Model file for the job. Use its own axes, mm. Face numbers are marked on the shaded views. A direction names the side the tool comes from. Round coordinates to 2 decimals unless told otherwise and drop trailing zeros. Order: outer loops, then holes, each group sorted by start corner. A loop starts at its lowest first (then second) coordinate and runs counter-clockwise, first axis right, second up. Notation, with made-up numbers: (6, 70.5) - (36, 70.5) arc R8 cw to (36, 78.5) - close; hole circle Ø9 at (8.5, 76.25). An arc over 180 degrees is marked (long way). Put each result on its own line as item: value. Start each with the question number.
Item 1: Saw through at A-A on z = -3.5. List the corners of the cut face in (x, y), plus the area to 3 significant figures.
Item 2: Pin check, flat tips, straight feed: pin 1 Ø3 at (x, y) = (17.51, 2.54) entering from -Z; pin 2 Ø1.5 at (x, y) = (-4.5, 4) entering from +Z; pin 3 Ø3.5 at (x, y) = (16, 3) entering from -Z; pin 4 Ø0.7 at (y, z) = (9.5, -3) entering from +X. Stop position of each tip, or through.
Item 3: Probe probe 1 along X at (y, z) = (9.5, -6.25); probe 2 along X at (y, z) = (9, -3.25); probe 3 along Y at (x, z) = (9, 1). List the from-to ranges inside material, lowest first.
Item 4: Mould opens along Y. For the marked faces 6, 7 and 8 say: pulls with the +Y half, pulls with the -Y half, needs draft (parallel to the pull), parting line crosses it, or undercut.
Item 5: Saw through at C-C on z = 4. List the corners of the cut face in (x, y), plus the area to 3 significant figures.
Item 6: Which spindle directions (+Z, -Z, +X, -X, +Y, -Y) get a long thin tool onto all of the face, cutting with end or side? Do the marked faces 1, 2, 3, 4 and 5. Say none if no direction does.
Item 7: Saw through at B-B on x = 6.5. List the corners of the cut face in (y, z).
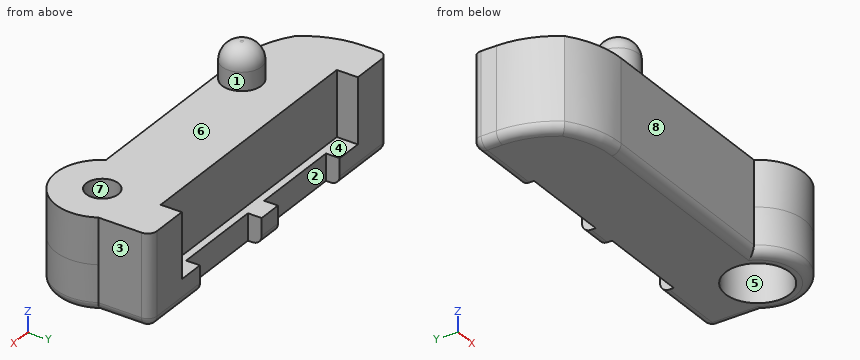
```python
from build123d import *

# Parameters (mm, degrees)
CROQUIS1_W              = 33
CROQUIS1_H              = 5
SALIENTE_EXTRUIR1_DEPTH = 8.5
CROQUIS2_W              = 5
CROQUIS2_H              = 8.5
SALIENTE_EXTRUIR2_DEPTH = 14
CORTAR_EXTRUIR1_REACH   = 34.055
CROQUIS5_R              = 5.070689822
SALIENTE_EXTRUIR3_DEPTH = 5
CROQUIS6_R              = 1.75
CORTAR_EXTRUIR2_DEPTH   = 5
SALIENTE_EXTRUIR4_START = 5
CROQUIS7_R              = 3.5
SALIENTE_EXTRUIR4_DEPTH = 5
SALIENTE_EXTRUIR5_DEPTH = 2.3
CROQUIS9_W              = 10
CROQUIS9_H              = 2.9
CORTAR_EXTRUIR3_DEPTH   = 1.5
CHAFL_N1_SIZE           = 4
REDONDEO1_R             = 10
REDONDEO3_R             = 1
REDONDEO4_R             = 1
REDONDEO5_R             = 1
REDONDEO6_R             = 1
REDONDEO7_R             = 1
CROQUIS10_R             = 2.15
SALIENTE_EXTRUIR6_DEPTH = 4
REDONDEO8_R             = 2


with BuildPart() as part:
    # Croquis1 → Saliente-Extruir1 (new body)
    with BuildSketch(Plane(origin=(0, 0, 0), x_dir=(1, 0, 0), z_dir=(0, 1, 0))):
        Rectangle(CROQUIS1_W, CROQUIS1_H)
    extrude(amount=SALIENTE_EXTRUIR1_DEPTH)

    # Croquis2 → Saliente-Extruir2 (add)
    with BuildSketch(Plane(origin=(16.5, 0, 0), x_dir=(0, 0, -1), z_dir=(1, 0, 0))):
        with Locations((0, 4.25)):
            Rectangle(CROQUIS2_W, CROQUIS2_H)
    extrude(amount=SALIENTE_EXTRUIR2_DEPTH)

    # Croquis4 → Cortar-Extruir1 (cut, up to next)
    with BuildSketch(Plane(origin=(0, 0, -2.5), x_dir=(-1, 0, 0), z_dir=(0, 0, -1)), mode=Mode.PRIVATE) as cortar_extruir1_sk1:
        Polygon((-21.898835729, 8.5), (-21.898835729, 2.753380039), (-21.898835729, 0), (-30.5, 0), (-30.5, 8.5), align=None)
    cortar_extruir1_tool1 = extrude(cortar_extruir1_sk1.sketch, amount=-CORTAR_EXTRUIR1_REACH, mode=Mode.PRIVATE) & part.part
    add(cortar_extruir1_tool1.solids().sort_by_distance((26.199418, 4.25, -2.5))[0], mode=Mode.SUBTRACT)

    # Croquis5 → Saliente-Extruir3 (add)
    with BuildSketch(Plane(origin=(0, 0, -2.5), x_dir=(-1, 0, 0), z_dir=(0, 0, -1))):
        with Locations((-17.511321809, 2.541971061)):
            Circle(CROQUIS5_R)
    extrude(amount=-SALIENTE_EXTRUIR3_DEPTH)

    # Croquis6 → Cortar-Extruir2 (cut)
    with BuildSketch(Plane(origin=(0, 0, -2.5), x_dir=(-1, 0, 0), z_dir=(0, 0, -1))):
        with Locations((-17.511321809, 2.541971061)):
            Circle(CROQUIS6_R)
    extrude(amount=-CORTAR_EXTRUIR2_DEPTH, mode=Mode.SUBTRACT)

    # Croquis7 → Saliente-Extruir4 (add)
    with BuildSketch(Plane(origin=(0, 0, -2.5), x_dir=(-1, 0, 0), z_dir=(0, 0, -1)).offset(SALIENTE_EXTRUIR4_START)):
        with BuildLine():
            Line((-21.898835729, 8.5), (-21.898835729, 5.083942123))
            ThreePointArc((-21.898835729, 5.083942123), (-20.05329287, -1.845542858), (-13.123807889, 0))
            Line((-13.123807889, 0), (16.5, 0))
            Line((16.5, 0), (16.5, 8.5))
            Line((16.5, 8.5), (-21.898835729, 8.5))
        make_face()
        with Locations((-17.511321809, 2.541971061)):
            Circle(CROQUIS7_R, mode=Mode.SUBTRACT)
    extrude(amount=-SALIENTE_EXTRUIR4_DEPTH)

    # Croquis8 → Saliente-Extruir5 (add)
    with BuildSketch(Plane(origin=(0, 8.5, 0), x_dir=(1, 0, 0), z_dir=(0, 1, 0))):
        Polygon((-16.5, -2.5), (-11.620504371, -2.5), (-11.620504371, -2.1), (-11.620504371, 4.6), (16.879495629, 4.6), (16.879495629, -2.1), (16.879495629, -2.5), (21.898835729, -2.5), (21.898835729, 7.5), (-16.5, 7.5), align=None)
    extrude(amount=SALIENTE_EXTRUIR5_DEPTH)

    # Croquis9 → Cortar-Extruir3 (cut)
    with BuildSketch(Plane(origin=(0, 10.8, 0), x_dir=(1, 0, 0), z_dir=(0, 1, 0))):
        with Locations((8.949495629, 6.05)):
            Rectangle(CROQUIS9_W, CROQUIS9_H)
        with Locations((-3.690504371, 6.05)):
            Rectangle(CROQUIS9_W, CROQUIS9_H)
    extrude(amount=-CORTAR_EXTRUIR3_DEPTH, mode=Mode.SUBTRACT)

    # Chaflán1
    chafl_n1_edges = [part.edges().sort_by_distance(p)[0] for p in [
        (-16.5, 0, -2.5),
    ]]
    chamfer(chafl_n1_edges, length=CHAFL_N1_SIZE)

    # Redondeo1
    # the kernel refuses this fillet: 10 mm, written as the material it takes off along each edge
    with BuildSketch(Plane(origin=(-12.5, 0, 12.855339059), x_dir=(-0.7071067811865476, 0.7071067811865477, 0), z_dir=(0, 0, -1)), Plane(origin=(-16.5, 4, 12.855339059), x_dir=(0, 1, 0), z_dir=(0, 0, -1))) as redondeo1_piece_1:
        with BuildLine():
            CenterArc((REDONDEO1_R * 0.414213562373, REDONDEO1_R), REDONDEO1_R, 225, 45)
            Line((-REDONDEO1_R * 0.292893218813, REDONDEO1_R * 0.292893218813), (0, 0))
            Line((0, 0), (REDONDEO1_R * 0.414213562373, 0))
        make_face()
    extrude(amount=30.710678119, mode=Mode.SUBTRACT)

    # Redondeo3
    redondeo3_edges = [part.edges().sort_by_distance(p)[0] for p in [
        (-16.5, 9.471067812, -7.5),
        (-15.970669758, 4.931775157, -7.5),
        (-11.568224843, 0.529330242, -7.5),
        (2.382971757, 0, -7.5),
    ]]
    fillet(redondeo3_edges, radius=REDONDEO3_R)

    # Redondeo4
    redondeo4_edges = [part.edges().sort_by_distance(p)[0] for p in [
        (19.565273177, -2.094102606, -7.5),
        (21.898835729, 7.941971061, -7.5),
    ]]
    fillet(redondeo4_edges, radius=REDONDEO4_R)

    # Redondeo5
    redondeo5_edges = [part.edges().sort_by_distance(p)[0] for p in [
        (17.424165679, 10.8, -7.5),
        (21.60594251, 10.8, -7.207106781),
        (21.898835729, 10.8, -2),
    ]]
    fillet(redondeo5_edges, radius=REDONDEO5_R)

    # Redondeo6
    redondeo6_edges = [part.edges().sort_by_distance(p)[0] for p in [
        (-12.095252185, 10.8, -7.5),
        (-16.5, 10.8, -2),
        (-16.207106781, 10.8, -7.207106781),
    ]]
    fillet(redondeo6_edges, radius=REDONDEO6_R)

    # Redondeo7
    redondeo7_edges = [part.edges().sort_by_distance(p)[0] for p in [
        (2.629495629, 10.8, -7.5),
    ]]
    fillet(redondeo7_edges, radius=REDONDEO7_R)

    # Croquis10 → Saliente-Extruir6 (add)
    with BuildSketch(Plane.XY.offset(2.5)):
        with Locations((-5.503268941, 2.252495098)):
            Circle(CROQUIS10_R)
    extrude(amount=SALIENTE_EXTRUIR6_DEPTH)

    # Redondeo8
    redondeo8_edges = [part.edges().sort_by_distance(p)[0] for p in [
        (-7.653268941, 2.252495098, 6.5),
    ]]
    fillet(redondeo8_edges, radius=REDONDEO8_R)


solid = part.part
```
Results found:
1. outline: (-16.5, 8.14) arc R10 ccw to (-14.44, 2.06) arc R10 ccw to (-8.36, 0) - (13.12, 0) arc R5.07 ccw to (21.9, 5.08) - (21.9, 9.8) arc R1 ccw to (20.9, 10.8) - (16.88, 10.8) - (16.88, 8.5) - (-11.62, 8.5) - (-11.62, 10.8) - (-15.5, 10.8) arc R1 ccw to (-16.5, 9.8) - close; hole circle Ø7 at (17.51, 2.54)
1. area: 316 mm²
2. pin 1: passes through
2. pin 2: stops at z = 6.16
2. pin 3: stops at z = -2.5
2. pin 4: stops at x = 21.9
3. probe 1: x = -16.5 to -8.69, 1.31 to 3.95, 13.95 to 21.9
3. probe 2: x = -16.5 to -11.62, 16.88 to 21.9
3. probe 3: y = 0 to 8.5
4. face 6: needs draft
4. face 7: undercut
4. face 8: pulls with the -Y half
5. outline: circle Ø4.3 at (-5.5, 2.25)
5. area: 14.5 mm²
6. face 1: +Z
6. face 2: +Z, -Z, +Y
6. face 3: +Z, -Z, +X, +Y
6. face 4: +Z, +Y
6. face 5: -Z
7. outline: (0, -6.5) arc R1 ccw to (1, -7.5) - (9.3, -7.5) - (9.3, -4.6) - (8.5, -4.6) - (8.5, 2.5) - (0, 2.5) - close
